from build123d import *

# Parameters (mm, degrees)
F1_DEPTH = 25.4


with BuildPart() as f1:
    # F0 (on Top) → F1 (new body)
    with BuildSketch(Plane.XY):
        Polygon((-63.21651, 21.525792), (-27.295485, 57.446817), (-40.443493, 106.515849), (-89.512525, 119.663856), (-125.433549, 83.742832), (-112.285542, 34.6738), align=None)
        Polygon((-86.225523, 107.396598), (-49.423749, 97.535593), (-39.562743, 60.733819), (-66.503511, 33.79305), (-103.305285, 43.654056), (-113.166291, 80.45583), align=None, mode=Mode.SUBTRACT)
        Polygon((59.425539, -29.274208), (59.425539, 21.525792), (23.504515, 57.446817), (-27.295485, 57.446817), (-63.21651, 21.525792), (-63.21651, -29.274208), (-27.295485, -65.195232), (23.504515, -65.195232), align=None)
        Polygon((-40.443493, -114.264264), (-27.295485, -65.195232), (-63.21651, -29.274208), (-112.285542, -42.422215), (-125.433549, -91.491247), (-89.512525, -127.412272), align=None)
        Polygon((-113.166291, -88.204245), (-103.305285, -51.402471), (-66.503511, -41.541466), (-39.562743, -68.482234), (-49.423749, -105.284008), (-86.225523, -115.145014), align=None, mode=Mode.SUBTRACT)
        Polygon((108.494571, -42.422215), (59.425539, -29.274208), (23.504515, -65.195232), (36.652522, -114.264264), (85.721554, -127.412272), (121.642579, -91.491247), align=None)
        Polygon((35.771773, -68.482234), (62.712541, -41.541466), (99.514315, -51.402471), (109.375321, -88.204245), (82.434552, -115.145014), (45.632778, -105.284008), align=None, mode=Mode.SUBTRACT)
        Polygon((23.504515, 57.446817), (59.425539, 21.525792), (108.494571, 34.6738), (121.642579, 83.742832), (85.721554, 119.663856), (36.652522, 106.515849), align=None)
        Polygon((45.632778, 97.535593), (82.434552, 107.396598), (109.375321, 80.45583), (99.514315, 43.654056), (62.712541, 33.79305), (35.771773, 60.733819), align=None, mode=Mode.SUBTRACT)
    extrude(amount=F1_DEPTH)


solid = f1.part
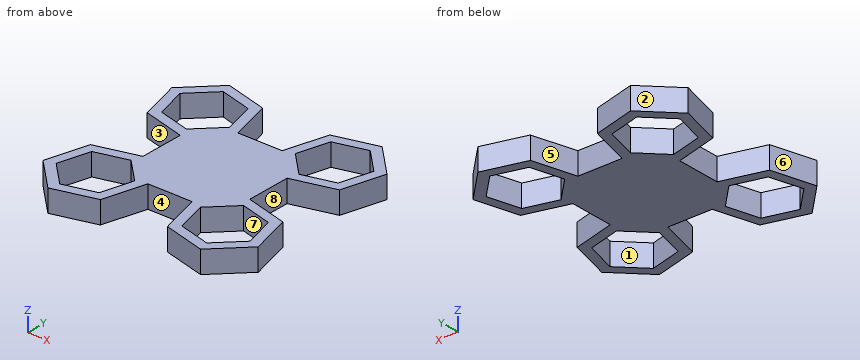
For this review, take the finished solid that the model builds, in its own axes (mm). Face numbers are marked on the shaded views. A direction names the side the tool comes from. Coordinates: 2 decimals unless noted, no trailing zeros. Loops run counter-clockwise (first coordinate to the right, second up) from the corner with the lowest first, then second, coordinate; pieces in that order, holes last. Notation, with made-up numbers: (25, 88.5) - (82, 88.5) arc R25 cw to (82, 102.5) - close; hole circle Ø7 at (34, 20.25). An arc over 180 degrees is marked (long way). Return JSON: item names as keys, results as strings.
Item 1: Insertion check: pin 1 (1 mm diameter, centred on y = 76, z = 10.5, fed in from -X); pin 2 (1.5 mm diameter, centred on y = 65.5, z = 19.5, fed in from -X); pin 3 (4 mm diameter, centred on y = -66, z = 20.5, fed in from -X). Each pin has a flat end and moves straight along its axis. Give the tip position at first contact, or say it passes through.
Determined:
{"pin 1": "stops at x = -123.49", "pin 2": "stops at x = -120.75", "pin 3": "stops at x = -119.14"}
Item 2: Take a section at B-B (x = 96). Give the boundary of the cut face in (y, z), then the cut area to 3 significant figures.
Determined:
{"outline": "(-117.13, 0) - (-101.58, 0) - (-101.58, 25.4) - (-117.13, 25.4) - close; (-50.46, 0) - (-39.07, 0) - (-39.07, 25.4) - (-50.46, 25.4) - close; (31.33, 0) - (42.71, 0) - (42.71, 25.4) - (31.33, 25.4) - close; (93.83, 0) - (109.39, 0) - (109.39, 25.4) - (93.83, 25.4) - close", "area": "1,370 mm2"}
Item 3: Mouldability with a two-part tool opening along X and no side actions: class the marked faces 6, 7 and 8 as pulls with the +X half, pulls with the -X half, needs draft (parallel to the pull), parting line crosses it, or undercut.
Determined:
{"face 6": "pulls with the -X half", "face 7": "undercut", "face 8": "pulls with the +X half"}
Item 4: For the marked faces 1, 2, 3, 4 and 5, list the 3-axis set-ups (+Z, -Z, +X, -X, +Y, -Y) from which the entire face can be reached by the end or side of a thin tool; tool diameter is ignored.
Determined:
{"face 1": "+Z, -Z", "face 2": "+Z, -Z, -X, +Y", "face 3": "+Z, -Z, -X", "face 4": "+Z, -Z, -Y", "face 5": "+Z, -Z, +Y"}
Item 5: Take a section at D-D (z = 17.5). State how many separate pieces and enclosed holes the cut face has, then the cut area to 3 significant figures.
Determined:
{"separate pieces": "1", "enclosed holes": "4", "area": "24,200 mm2"}
Item 6: For line 1 (Y direction, x = -93, z = 16.75); line 2 (Y direction, x = -102, z = 1); line 3 (X direction, y = 93.5, z = 22.25), list the stretches that pass through material, from the lowest coordinate up.
Determined:
{"line 1": "y = -123.92 to -108.37, -48.64 to -37.25, 29.51 to 40.89, 100.62 to 116.18", "line 2": "y = -114.92 to -99.37, -51.05 to -39.67, 31.92 to 43.3, 91.62 to 107.18", "line 3": "x = -115.68 to -100.12, -48.34 to -36.96, 33.16 to 44.55, 96.33 to 111.89"}
Item 7: Take a section at A-A (y = -72). Give the boundary of the cut face in (x, z), then the cut area to 3 significant figures.
Determined:
{"outline": "(-120.21, 0) - (-108.82, 0) - (-108.82, 25.4) - (-120.21, 25.4) - close; (-40.51, 0) - (-29.12, 0) - (-29.12, 25.4) - (-40.51, 25.4) - close; (25.33, 0) - (36.71, 0) - (36.71, 25.4) - (25.33, 25.4) - close; (105.03, 0) - (116.42, 0) - (116.42, 25.4) - (105.03, 25.4) - close", "area": "1,160 mm2"}
Item 8: Take a section at C-C (x = 50). Give the boundary of the cut face in (y, z), then the cut area to 3 significant figures.
Determined:
{"outline": "(-117.84, 0) - (-106.45, 0) - (-106.45, 25.4) - (-117.84, 25.4) - close; (-54.25, 0) - (46.51, 0) - (46.51, 25.4) - (-54.25, 25.4) - close; (98.71, 0) - (110.09, 0) - (110.09, 25.4) - (98.71, 25.4) - close", "area": "3,140 mm2"}
